The model under review builds one solid part; all positions refer to its coordinate system, in mm. Give positions to 0.01 mm unless a question says otherwise; leave off trailing zeros. Order: outer loops, then holes, each group sorted by start corner. A loop starts at its lowest first (then second) coordinate and runs counter-clockwise, first axis right, second up. Notation, with made-up numbers: (3, -35) -> (17, -35) arc R15 cw to (17, -11) -> close; hole circle Ø3 at (-39.75, -5.75). An arc over 180 degrees is marked (long way). Answer as a JSON object with one key per item and string values. Group by question number.
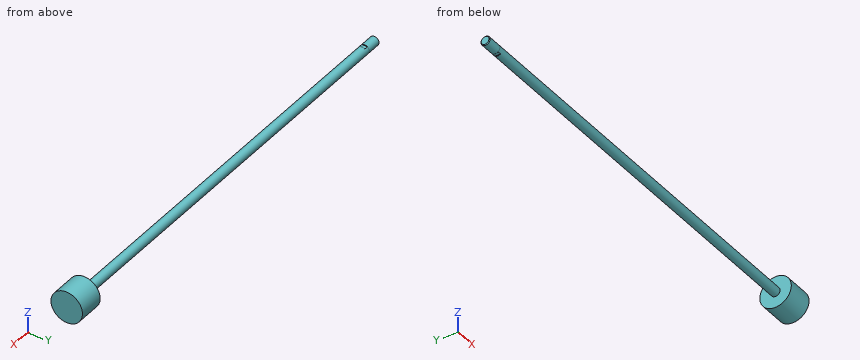
Autodesk Inventor part; units mm, degrees
ref_plane "rod_cp_XY" through (0, 0, 0) normal (1, 0, 0) x (0, 0, -1)
ref_plane "rod_cp_YZ" through (0, 0, 0) normal (0, 0, -1) x (0, 1, 0)
ref_plane "rod_cp_ZX" through (0, 0, 0) normal (0, 1, 0) x (1, 0, 0)
sketch "Sketch_1" plane through (0, 0, 0) normal (0, 0, 1) x (1, 0, 0)
  line L0 (368.1984, 0) -> (-3.175, 0)
  line L1 (-3.175, 0) -> (-3.175, 3.9624)
  line L2 (-3.175, 3.9624) -> (346.075, 3.9624)
  line L3 (346.075, 3.9624) -> (346.075, 13.5572)
  line L4 (346.075, 13.5572) -> (368.1984, 13.5572)
  line L5 (368.1984, 13.5572) -> (368.1984, 0)
  line L6 (368.1984, 0) -> (-3.175, 0)
revolve "Revolution1" add sketch "Sketch_1" angle 360 about axis through (368.1984, 0, 0) along (1, 0, 0)
sketch "Sketch_3" plane through (0, 0, 0) normal (0, 0, 1) x (1, 0, 0)
  line L0 (-3.175, 0) -> (-15.875, 0)
  line L1 (-15.875, 0) -> (-15.875, 3.3388)
  line L2 (-15.875, 3.3388) -> (-15.2451, 3.9688)
  line L3 (-15.2451, 3.9688) -> (-3.175, 3.9688)
  line L4 (-3.175, 3.9688) -> (-3.175, 0)
  line L5 (-3.175, 0) -> (-15.875, 0)
revolve "Revolution2" add sketch "Sketch_3" angle 360 about axis through (-3.175, 0, 0) along (1, 0, 0)
thread "Thread1"
sketch "Sketch_10" plane through (-3.175, 0, 0) normal (1, 0, 0) x (0, 0, -1)
  line L0 (-7.9248, 7.9248) -> (-7.9248, -7.9248)
  line L1 (-7.9248, -7.9248) -> (7.9248, -7.9248)
  line L2 (7.9248, -7.9248) -> (7.9248, 7.9248)
  line L3 (7.9248, 7.9248) -> (-7.9248, 7.9248)
  line L4 (-3.175, 3.9624) -> (-3.175, -3.9624)
  line L5 (-3.175, -3.9624) -> (3.175, -3.9624)
  line L6 (3.175, -3.9624) -> (3.175, 3.9624)
  line L7 (3.175, 3.9624) -> (-3.175, 3.9624)
extrude "Extrusion1" cut sketch "Sketch_10" along normal blind 3.175
ref_plane "rod_cp_XY" through (0, 0, 0) normal (1, 0, 0) x (0, 0, -1)
ref_plane "rod_cp_YZ" through (0, 0, 0) normal (0, 0, -1) x (0, 1, 0)
ref_plane "rod_cp_ZX" through (0, 0, 0) normal (0, 1, 0) x (1, 0, 0)
ref_plane "to_rod_clevis_XY" through (-15.875, 0, 0) normal (1, 0, 0) x (0, 0, -1)
ref_plane "to_rod_clevis_YZ" through (-15.875, 0, 0) normal (0, 0, -1) x (0, 1, 0)
ref_plane "to_rod_clevis_ZX" through (-15.875, 0, 0) normal (0, 1, 0) x (1, 0, 0)
ref_plane "rl2_XY" through (-3.175, 0, 0) normal (1, 0, 0) x (0, 0, -1)
ref_plane "rl2_YZ" through (-3.175, 0, 0) normal (0, 0, -1) x (0, 1, 0)
ref_plane "rl2_ZX" through (-3.175, 0, 0) normal (0, 1, 0) x (1, 0, 0)
ref_plane "rl1_XY" through (-15.875, 0, 0) normal (1, 0, 0) x (0, 0, -1)
ref_plane "rl1_YZ" through (-15.875, 0, 0) normal (0, 0, -1) x (0, 1, 0)
ref_plane "rl1_ZX" through (-15.875, 0, 0) normal (0, 1, 0) x (1, 0, 0)
ref_plane "thd1_XY" through (-15.875, 3.9688, 0) normal (1, 0, 0) x (0, 0, -1)
ref_plane "thd1_YZ" through (-15.875, 3.9688, 0) normal (0, 0, -1) x (0, 1, 0)
ref_plane "thd1_ZX" through (-15.875, 3.9688, 0) normal (0, 1, 0) x (1, 0, 0)
ref_plane "thd2_XY" through (-15.875, -3.9688, 0) normal (1, 0, 0) x (0, 0, -1)
ref_plane "thd2_YZ" through (-15.875, -3.9688, 0) normal (0, 0, -1) x (0, 1, 0)
ref_plane "thd2_ZX" through (-15.875, -3.9688, 0) normal (0, 1, 0) x (1, 0, 0)
ref_plane "dia1_XY" through (-3.175, 3.9624, 0) normal (1, 0, 0) x (0, 0, -1)
ref_plane "dia1_YZ" through (-3.175, 3.9624, 0) normal (0, 0, -1) x (0, 1, 0)
ref_plane "dia1_ZX" through (-3.175, 3.9624, 0) normal (0, 1, 0) x (1, 0, 0)
ref_plane "dia2_XY" through (-3.175, -3.9624, 0) normal (1, 0, 0) x (0, 0, -1)
ref_plane "dia2_YZ" through (-3.175, -3.9624, 0) normal (0, 0, -1) x (0, 1, 0)
ref_plane "dia2_ZX" through (-3.175, -3.9624, 0) normal (0, 1, 0) x (1, 0, 0)
ref_plane "wf1_XY" through (-3.175, 0, 0) normal (1, 0, 0) x (0, 0, -1)
ref_plane "wf1_YZ" through (-3.175, 0, 0) normal (0, 0, -1) x (0, 1, 0)
ref_plane "wf1_ZX" through (-3.175, 0, 0) normal (0, 1, 0) x (1, 0, 0)
ref_plane "wf2_XY" through (0, 0, 0) normal (1, 0, 0) x (0, 0, -1)
ref_plane "wf2_YZ" through (0, 0, 0) normal (0, 0, -1) x (0, 1, 0)
ref_plane "wf2_ZX" through (0, 0, 0) normal (0, 1, 0) x (1, 0, 0)
ref_plane "hh1_XY" through (395.9606, 0, 0) normal (0, 0, 1) x (1, 0, 0)
ref_plane "hh1_YZ" through (395.9606, 0, 0) normal (1, 0, 0) x (0, 1, 0)
ref_plane "hh1_ZX" through (395.9606, 0, 0) normal (0, 1, 0) x (0, 0, 1)
ref_plane "hh2_XY" through (402.3614, 0, 0) normal (0, 0, 1) x (1, 0, 0)
ref_plane "hh2_YZ" through (402.3614, 0, 0) normal (1, 0, 0) x (0, 1, 0)
ref_plane "hh2_ZX" through (402.3614, 0, 0) normal (0, 1, 0) x (0, 0, 1)
ref_plane "dia12_XY" through (0, 0, 14.1351) normal (1, 0, 0) x (0, 0, -1)
ref_plane "dia12_YZ" through (0, 0, 14.1351) normal (0, 0, -1) x (0, 1, 0)
ref_plane "dia12_ZX" through (0, 0, 14.1351) normal (0, 1, 0) x (1, 0, 0)
ref_plane "dia22_XY" through (0, 0, -14.1351) normal (1, 0, 0) x (0, 0, -1)
ref_plane "dia22_YZ" through (0, 0, -14.1351) normal (0, 0, -1) x (0, 1, 0)
ref_plane "dia22_ZX" through (0, 0, -14.1351) normal (0, 1, 0) x (1, 0, 0)
ref_plane "wfw1_XY" through (-3.175, 0, -3.175) normal (0, 1, 0) x (1, 0, 0)
ref_plane "wfw1_YZ" through (-3.175, 0, -3.175) normal (1, 0, 0) x (0, 0, -1)
ref_plane "wfw1_ZX" through (-3.175, 0, -3.175) normal (0, 0, -1) x (0, 1, 0)
ref_plane "wfw2_XY" through (-3.175, 0, 3.175) normal (0, 1, 0) x (1, 0, 0)
ref_plane "wfw2_YZ" through (-3.175, 0, 3.175) normal (1, 0, 0) x (0, 0, -1)
ref_plane "wfw2_ZX" through (-3.175, 0, 3.175) normal (0, 0, -1) x (0, 1, 0)
properties part number "0912-DX0_rod"
1. For probe 1 along X at (y, z) = (-2.5, 10.25) (3 decimals); probe 2 along Z at (x, y) = (177, 0.25); probe 3 along Z at (x, y) = (81.5, 2.25), list the stretches that pass through material, from the lowest coordinate up. Write a range as [from, to].
2. Take a section at B-B on x = 87.5. Give the boundary of the cut face in (y, z).
3. For pin 1 (10 mm diameter, centred on y = -3.5, z = 8, fed in from -X); pin 2 (5 mm diameter, centred on y = -4, z = 11, fed in from -X) (3 decimals); pin 3 (1 mm diameter, centred on x = -1, y = 0, fed in from +Z) (3 decimals); pin 4 (10 mm diameter, centred on y = -2, z = -8, fed in from -X) (3 decimals), all flat-tipped, find the tip position at first contact; note any pin that passes through.
4. Take a section at C-C on y = 8. Give the boundary of the cut face in (x, z) (3 decimals), plus the area to 3 significant figures.
5. Take a section at A-A on z = 0. Give the boundary of the cut face in (x, y) (3 decimals), plus the area to 3 significant figures.
Checks:
{
 "1": {"probe 1": "x = [346.075, 368.198]", "probe 2": "z = [-3.95, 3.95]", "probe 3": "z = [-3.26, 3.26]"},
 "2": {"outline": "circle Ø7.92 at (0, 0)"},
 "3": {"pin 1": "stops at x = -15.48", "pin 2": "stops at x = 346.075", "pin 3": "stops at z = 3.175", "pin 4": "stops at x = -15.875"},
 "4": {"outline": "(346.075, -10.945) -> (368.198, -10.945) -> (368.198, 10.945) -> (346.075, 10.945) -> close", "area": "484 mm2"},
 "5": {"outline": "(-15.875, -3.339) -> (-15.245, -3.969) -> (-3.175, -3.969) -> (-3.175, -3.962) -> (346.075, -3.962) -> (346.075, -13.557) -> (368.198, -13.557) -> (368.198, 13.557) -> (346.075, 13.557) -> (346.075, 3.962) -> (-3.175, 3.962) -> (-3.175, 3.969) -> (-15.245, 3.969) -> (-15.875, 3.339) -> close", "area": "3,470 mm2"}
}
